Could you check a few things on this drawing? It's one solid part, dimensions in mm from its lowest x, y, z. A direction names the side the tool comes from. Coordinates: 2 decimals unless noted, no trailing zeros. Order: outer loops, then holes, each group sorted by start corner. A loop starts at its lowest first (then second) coordinate and runs counter-clockwise, first axis right, second up.
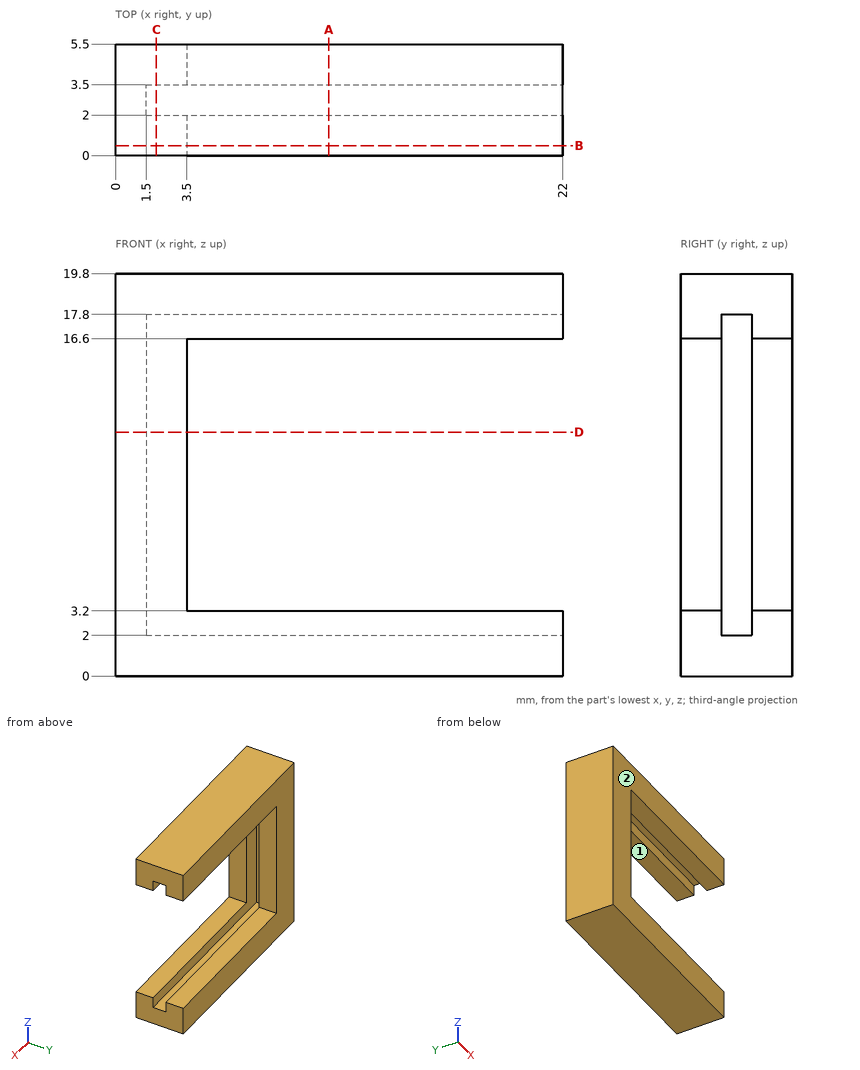
Q1. Will this pin go through, and if not, where does the flat tip stop? pin 1 (1.6 mm diameter, centred on y = 4.5, z = 10, fed in from +X).
Q2. If we section it at C-C on x = 2: Write out the boundary of the cut face in (y, z).
Q3. If we section it at D-D on z = 12: Write out the boundary of the cut face in (x, y), then the cut area to 4 significant figures.
Q4. I need wall thicknesses on L1, parallel to Z at x = 6, y = 1.85; L2, parallel to Y at x = 3.25, z = 11.5; L3, parallel to Z at x = 19, y = 2.9. Which ranges of each line are inside material? Lowest first, please.
Q5. If we section it at A-A on x = 10.5: Write out the boundary of the cut face in (y, z), then the cut area to 3 significant figures.
Q6. If we section it at B-B on y = 0.5: Write out the boundary of the cut face in (x, z).
Q7. For the marked faces 1 and 2, which set-ups out of +Z, -Z, +X, -X, +Y, -Y let a thin tool reach every point of the face, with its end or its side?
Reply:
1. pin 1: stops at x = 3.5
2. outline: (0, 0) - (5.5, 0) - (5.5, 19.8) - (0, 19.8) - close; hole (2, 2) - (3.5, 2) - (3.5, 17.8) - (2, 17.8) - close
3. outline: (0, 0) - (3.5, 0) - (3.5, 2) - (1.5, 2) - (1.5, 3.5) - (3.5, 3.5) - (3.5, 5.5) - (0, 5.5) - close
3. area: 16.25 mm2
4. L1: z = 0 to 3.2, 16.6 to 19.8
4. L2: y = 0 to 2, 3.5 to 5.5
4. L3: z = 0 to 2, 17.8 to 19.8
5. outline: (0, 0) - (5.5, 0) - (5.5, 3.2) - (3.5, 3.2) - (3.5, 2) - (2, 2) - (2, 3.2) - (0, 3.2) - close; (0, 16.6) - (2, 16.6) - (2, 17.8) - (3.5, 17.8) - (3.5, 16.6) - (5.5, 16.6) - (5.5, 19.8) - (0, 19.8) - close
5. area: 31.6 mm2
6. outline: (0, 0) - (22, 0) - (22, 3.2) - (3.5, 3.2) - (3.5, 16.6) - (22, 16.6) - (22, 19.8) - (0, 19.8) - close
7. face 1: +X, +Y, -Y
7. face 2: +Z, -Z, +X, -X, -Y
